For this review, take the finished solid that the model builds, in its own axes (mm). A direction names the side the tool comes from. Round coordinates to 2 decimals unless told otherwise and drop trailing zeros. Loops run counter-clockwise (first coordinate to the right, second up) from the corner with the lowest first, then second, coordinate; pieces in that order, holes last.
1. To check wall thickness, follow line 1 along Y through (x, z) = (38.5, 4); line 2 along Y through (x, z) = (29.5, 9); line 3 along Z through (x, y) = (19, 6). State the ranges of each line that lie inside material, in increasing order.
2. Consider section D-D on x = 27.5. State the section outline as (y, z) points.
3. Tool access review of faces 1 (the flat face through (0, 0, 0)), 2 (the cylindrical face through (35.77, 34.99, 22.78)), 3 (the cylindrical face through (34.23, -34.99, 22.78)): name each direction out of +Z, -Z, +X, -X, +Y, -Y from which nothing blocks a thin tool from reaching the whole face with its end or side.
4. Consider section B-B on y = 30. State the section outline as (x, z) points, then the cut area to 3 significant figures.
5. Clearance check with flat-ended pins moving along their axes: pin 1 Ø1 at (x, z) = (18, -6) entering from -Y; pin 2 Ø6 at (x, z) = (22, 8) entering from +Y; pin 3 Ø8 at (x, z) = (19.5, -10) entering from -Y. State where each tip first meets the part, or that it passes through.
6. Consider section A-A on z = 28. State the section outline as (x, y) points.
7. Consider section C-C on x = 35. State the section outline as (y, z) points.
from build123d import *
from build123d.topology import SkipClean

# Parameters (mm, degrees)
SKETCH_1_R      = 35
EXTRUDE_1_DEPTH = 70
SKETCH_2_R      = 35
EXTRUDE_2_DEPTH = 32


with BuildPart() as part:
    # 草图1 → 凸台-拉伸1 (new body)
    with BuildSketch(Plane(origin=(0, 0, 0), x_dir=(0, 0, -1), z_dir=(1, 0, 0))):
        Circle(SKETCH_1_R)
    extrude(amount=EXTRUDE_1_DEPTH)

    # 草图2 → 凸台-拉伸2 (add)
    with SkipClean():  # the faces are left unmerged after this step: merging them gives an invalid solid
        with BuildSketch(Plane.XY.offset(35)):
            with Locations((35, 0)):
                Circle(SKETCH_2_R)
        extrude(amount=-EXTRUDE_2_DEPTH)


solid = part.part
Resolved:
1. line 1: y = -34.82 to 34.82
1. line 2: y = -34.57 to 34.57
1. line 3: z = -34.48 to 35
2. outline: (-34.19, 7.5) arc R35 ccw (long way) to (34.19, 7.5) - (34.19, 35) - (-34.19, 35) - close
3. face 1: +Z, -Z, -X, +Y, -Y
3. face 2: +Z, +Y
3. face 3: +Z, -Y
4. outline: (0, -18.03) - (70, -18.03) - (70, 18.03) - (53.03, 18.03) - (53.03, 35) - (16.97, 35) - (16.97, 18.03) - (0, 18.03) - close
4. area: 3,140 mm2
5. pin 1: stops at y = -34.57
5. pin 2: stops at y = 34.64
5. pin 3: stops at y = -34.48
6. outline: (0, -21) - (7, -21) arc R35 ccw to (63, -21) - (70, -21) - (70, 21) - (63, 21) arc R35 ccw to (7, 21) - (0, 21) - close
7. outline: (-35, 3) - (-34.87, 3) arc R35 ccw (long way) to (34.87, 3) - (35, 3) - (35, 35) - (-35, 35) - close
